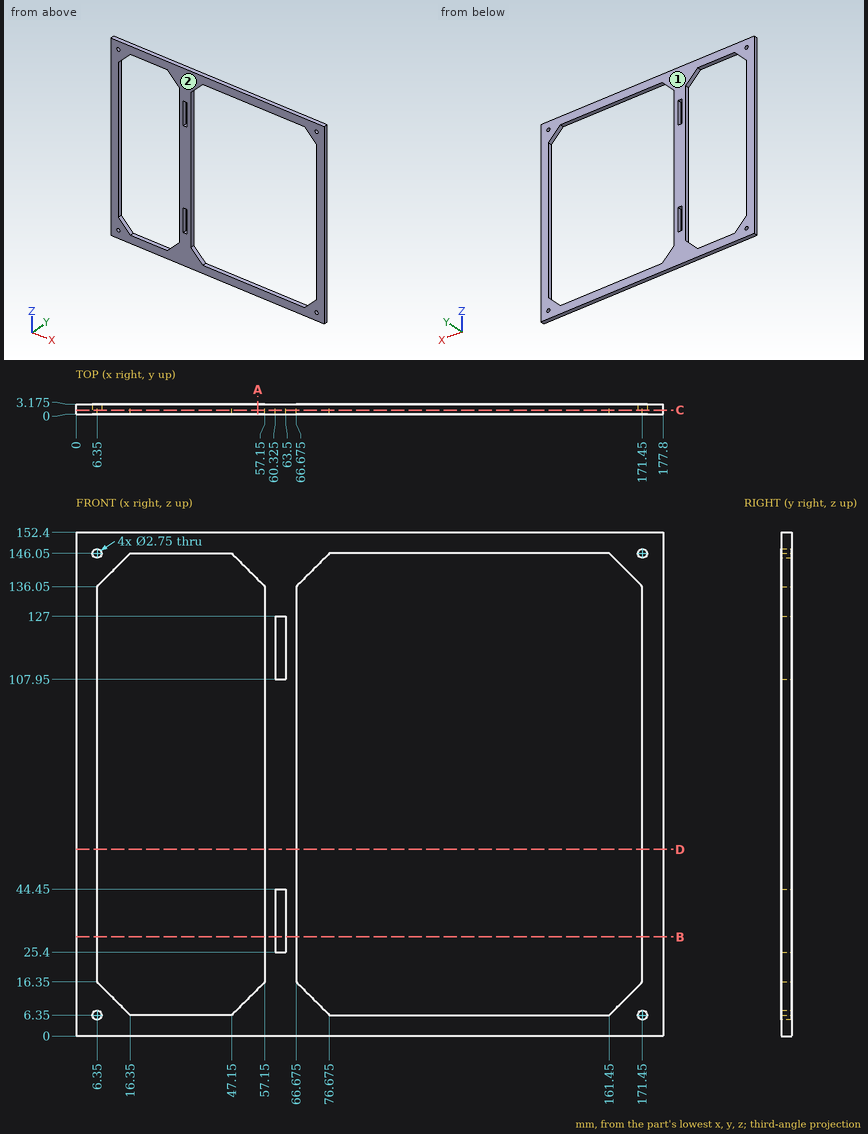
Source: three-view drawing plus pictorial views. Frame: mm from the lowest corner of the part. Round coordinates to 2 decimals unless told otherwise and drop trailing zeros. Loops run counter-clockwise (first coordinate to the right, second up) from the corner with the lowest first, then second, coordinate; pieces in that order, holes last. Notation, with made-up numbers: M 4,11.25 L 48,11.25 A16 cw 48,19.25 Z; hole C 45,48.5 d11. An arc over 180 degrees is marked long. Put each result on its own line as item: value. Start each with the question number.
(1) Section query B-B (z = 30). Return loops of the section in (x, y) (3 decimals).
(2) Section query D-D (z = 56.5). Return loops of the section in (x, y) (3 decimals), then the cut area to 3 significant figures.
(3) Section query C-C (y = 1.35). State how many separate pieces and enclosed holes the cut face has, then the cut area to 3 significant figures.
(4) Draft query along Y for the marked faces 1 and 2. Return one class per face: +Y half, -Y half, draft (parallel to the pull), parting line (faces both ways), or undercut.
(5) Material intervals for line 1 along X through (y, z) = (1.3, 50) (3 decimals); line 2 along X through (y, z) = (1.65, 125) (3 decimals); line 3 along Z through (x, y) = (86, 3.05), sorted ascending. Write a range as [from, to].
(6) Section query A-A (x = 55). Return loops of the section in (y, z) (3 decimals).
Findings below:
1. outline: M 0,0 L 6.35,0 L 6.35,3.175 L 0,3.175 Z; M 57.15,0 L 60.325,0 L 60.325,3.175 L 57.15,3.175 Z; M 63.5,0 L 66.675,0 L 66.675,3.175 L 63.5,3.175 Z; M 171.45,0 L 177.8,0 L 177.8,3.175 L 171.45,3.175 Z
2. outline: M 0,0 L 6.35,0 L 6.35,3.175 L 0,3.175 Z; M 57.15,0 L 66.675,0 L 66.675,3.175 L 57.15,3.175 Z; M 171.45,0 L 177.8,0 L 177.8,3.175 L 171.45,3.175 Z
2. area: 70.6 mm2
3. separate pieces: 1
3. enclosed holes: 8
3. area: 5,620 mm2
4. face 1: +Y half
4. face 2: -Y half
5. line 1: x = [0, 6.35], [57.15, 66.675], [171.45, 177.8]
5. line 2: x = [0, 6.35], [57.15, 60.325], [63.5, 66.675], [171.45, 177.8]
5. line 3: z = [0, 6.35], [146.05, 152.4]
6. outline: M 0,0 L 3.175,0 L 3.175,14.2 L 0,14.2 Z; M 0,138.2 L 3.175,138.2 L 3.175,152.4 L 0,152.4 Z
